The listing builds one solid part. Answer for the finished solid, in the listing's coordinates (mm). Give positions to 0.01 mm unless a question says otherwise; leave off trailing zeros. Loops run counter-clockwise (first coordinate to the right, second up) from the corner with the lowest first, then second, coordinate; pieces in that order, holes last.
Item 1: Section D-D, the plane x = -17.25 is taken. Give the vertices of the cut face in (y, z).
Item 2: The mould has two halves that part along Y. Classify faces 1 (the face through (-20, 0, 0)), 2 (the face through (0, -12.9, 6.5)), 3 (the face through (-9.367, 5.181, -16.453)), 4 (the face through (-8.875, 13.821, 1.815)): pulls with the +Y half, pulls with the -Y half, needs draft (parallel to the pull), parting line crosses it, or undercut.
Item 3: Each of these flat-tipped pins is pushed along its axis until it touches: pin 1 Ø1.5 at (x, y) = (-3, -5.5) entering from +Z; pin 2 Ø10 at (x, y) = (-20.5, -9) entering from +Z; pin 3 Ø8 at (x, z) = (-10.5, -5.5) entering from +Y. Where does it stop, or does it pass through?
Item 4: Section A-A, the plane z = 0 is taken. Give the vertices of the cut face in (x, y).
Item 5: Consider line 1 along X through (y, z) = (0.5, 5); line 2 along Z through (x, y) = (-9.25, 5); line 3 along Z through (x, y) = (-4.5, 9). Determine where each line is inside the solid, lowest interval first.
Item 6: Section C-C, the plane x = -1.5 is taken. Give the vertices of the cut face in (y, z), and give its area (3 significant figures).
Item 7: Section B-B, the plane x = -20.5 is taken. Give the vertices of the cut face in (y, z), and give its area (3 significant figures).
Autodesk Inventor part; units mm, degrees
ref_plane "YZ Plane" through (0, 0, 0) normal (1, 0, 0) x (0, 1, 0)
ref_plane "XZ Plane" through (0, 0, 0) normal (0, 1, 0) x (-1, 0, 0)
ref_plane "XY Plane" through (0, 0, 0) normal (0, 0, 1) x (1, 0, 0)
sketch "Sketch1" plane through (0, 0, 0) normal (0, 1, 0) x (-1, 0, 0)
  line L0 (23, 0) -> (23, -17.25)
  line L1 (23, -17.25) -> (0, -17.25)
  line L2 (0, -17.25) -> (0, -14.25)
  line L3 (0, -14.25) -> (20, -13.5516)
  line L4 (20, -13.5516) -> (20, 0)
  line L5 (20, 0) -> (23, 0)
  line L6 (0, 0) -> (20, 0) construction
  dimension "d0" = 2
  dimension "d1" = 28.5
  dimension "d2" = 20
  dimension "d3" = 3
  dimension "d4" = 3
  dimension "d14" = 27.1032
revolve "Revolution1" add sketch "Sketch1" angle 360 about axis through (0, 0, 0) along (-1, 0, 0)
chamfer "Chamfer1" distance 4 angle 45 1 edges at (-23, 0, 17.25)
chamfer "Chamfer2" distance 2 angle 45 1 edges at (-20, 0, 13.5516)
properties part number "vacum_cap"
Worked answers:
1. outline: circle Ø34.5 at (0, 0); hole circle Ø27.3 at (0, 0)
2. face 1: undercut
2. face 2: needs draft
2. face 3: parting line crosses it
2. face 4: undercut
3. pin 1: stops at z = 16.58
3. pin 2: stops at z = 16.72
3. pin 3: stops at y = 17.18
4. outline: (-23, -13.25) - (-19, -17.25) - (0, -17.25) - (0, -14.25) - (-18, -13.62) - (-20, -11.55) - (-20, 11.55) - (-18, 13.62) - (0, 14.25) - (0, 17.25) - (-19, 17.25) - (-23, 13.25) - close
5. line 1: x = -23 to -20
5. line 2: z = -16.51 to -13, 13 to 16.51
5. line 3: z = -14.72 to -10.84, 10.84 to 14.72
6. outline: circle Ø34.5 at (0, 0); hole circle Ø28.4 at (0, 0)
6. area: 302 mm2
7. outline: circle Ø31.5 at (0, 0)
7. area: 779 mm2
